Check sheet for the modelled part. Datum: model origin and axes. Units: mm. A direction names the side the tool comes from. Round coordinates to 2 decimals unless told otherwise and drop trailing zeros. Order: outer loops, then holes, each group sorted by start corner. A loop starts at its lowest first (then second) coordinate and runs counter-clockwise, first axis right, second up. Notation, with made-up numbers: (34, 77) -> (77, 77) arc R20 ccw to (77, 98) -> close; hole circle Ø6 at (35.5, 69.25). An arc over 180 degrees is marked (long way). Answer in a Markdown table with one row per item. Add a question column.
1. Material ranges on L1, parallel to Z at x = -19, y = 18; L2, parallel to Z at x = 0.5, y = 28.5; L3, parallel to X at y = 30.5, z = 0.5, recorded low to high. Write a range as from..to.
2. Sectioned sample at B-B, the plane x = -10. Record the boundary of the cut face in (y, z).
3. Sectioned sample at C-C, the plane z = -1.5. Record the boundary of the cut face in (x, y).
4. Depth check by flat-ended pin: P1, Ø1.5, axis at x = -27.5, y = 34.5, coming from the -Z side; P2, Ø12, axis at x = -19, y = 18.5, coming from the +Z side; P3, Ø2, axis at y = 18, z = -1.5, coming from the +X side. Enter the tip coordinate at first touch or a pass-through.
5. Access from +Z, -Z, +X, -X, +Y, -Y to the whole of each face (thin tool, end or side, straight path). Record for faces 1 (the cylindrical face through (3.447, 19.72, -0.138)), 2 (the flat face through (-21, 20, -1)), 3 (the flat face through (-20, 20, 1)).
Autodesk Inventor part; units mm, degrees
ref_plane "YZ Plane" through (0, 0, 0) normal (1, 0, 0) x (0, 1, 0)
ref_plane "XZ Plane" through (0, 0, 0) normal (0, 1, 0) x (-1, 0, 0)
ref_plane "XY Plane" through (0, 0, 0) normal (0, 0, 1) x (1, 0, 0)
sketch "Sketch1" plane through (0, 0, 0) normal (0, 1, 0) x (-1, 0, 0)
  point P0 (0, 0)
sketch "Sketch2" plane through (0, 0, 0) normal (0, 1, 0) x (-1, 0, 0)
  circle A0 centre (0, 0) radius 3.45
  dimension "d0" = 6.9
extrude "Extrusion1" add sketch "Sketch2" along normal blind 40
sketch "Sketch3" plane through (0, 40, 0) normal (0, 1, 0) x (1, 0, 0)
  line L0 (0, 0.9998) -> (-40, 0.9998)
  line L1 (-40, 0.9998) -> (-40, -1.0002)
  line L2 (-40, -1.0002) -> (0, -1.0002)
  line L3 (0, -1.0002) -> (0, 0.9998)
  point P0 (0, 0)
  dimension "d3" = 40
  dimension "d4" = 2
extrude "Extrusion2" add sketch "Sketch3" against normal blind 40
chamfer "Chamfer1" distance 2 angle 45 1 edges at (-40, 20, 1.0002)
fillet "Fillet1" radius 4 1 edges at (-38.0005, 20, 1.0002)
properties part number "scoop"
Answer key:
| question | item | result |
|---|---|---|
| 1 | L1 | z = -1..1 |
| 1 | L2 | z = -3.41..3.41 |
| 1 | L3 | x = -38.28..3.41 |
| 2 | outline | (0, -1) -> (40, -1) -> (40, 1) -> (0, 1) -> close |
| 3 | outline | (-3.11, 0) -> (3.11, 0) -> (3.11, 40) -> (-3.11, 40) -> close |
| 4 | P1 | stops at z = -1 |
| 4 | P2 | stops at z = 1 |
| 4 | P3 | stops at x = 3.41 |
| 5 | face 1 | +Y, -Y |
| 5 | face 2 | -Z, -X, +Y, -Y |
| 5 | face 3 | +Z, -X, +Y, -Y |
